Input: dimensioned drawing with shaded views. Units: mm. Origin: part minimum x, y, z. A direction names the side the tool comes from. Coordinates: 2 decimals unless noted, no trailing zeros. Loops run counter-clockwise (first coordinate to the right, second up) from the corner with the lowest first, then second, coordinate; pieces in that order, holes last.
(1) Section C-C, the plane z = 22.5. Return loops of the section in (x, y), then the cut area to 3 significant figures.
(2) Set-up query: the marked faces 5 and 6. Return all of +Z, -Z, +X, -X, +Y, -Y with unobstructed straight access to the full face (end or side cutting, diameter ignored); none if empty.
(3) Section A-A, the plane y = 7. Return loops of the section in (x, z).
(4) Line query: L1, parallel to Y at x = 27.5, z = 11.75; L2, parallel to Z at x = 47, y = 9.5; L3, parallel to Y at x = 45, z = 25.9. Output: solid intervals per line, ascending.
(5) Contact query for flat-ended pins moving along their axis: P1, Ø8, axis at x = 20.5, y = 9.5, coming from the -Z side; P2, Ø4, axis at x = 15.5, y = 12, coming from the -Z side; P3, Ø0.8, axis at x = 7, y = 1, coming from the -Z side; P4, Ø8, axis at x = 25, z = 5, coming from the -Y side. Output: stop coordinate, or through.
(6) Section B-B, the plane x = 5. Return loops of the section in (y, z), then the cut area to 3 significant figures.
(7) Mould query, pull axis Y, two halves, no side actions, for the marked faces 1, 2, 3 and 4. Classes: released by +Y, released by -Y, zero draft, split by the parting line, or undercut.
(8) Section D-D, the plane x = 25. Return loops of the section in (y, z).
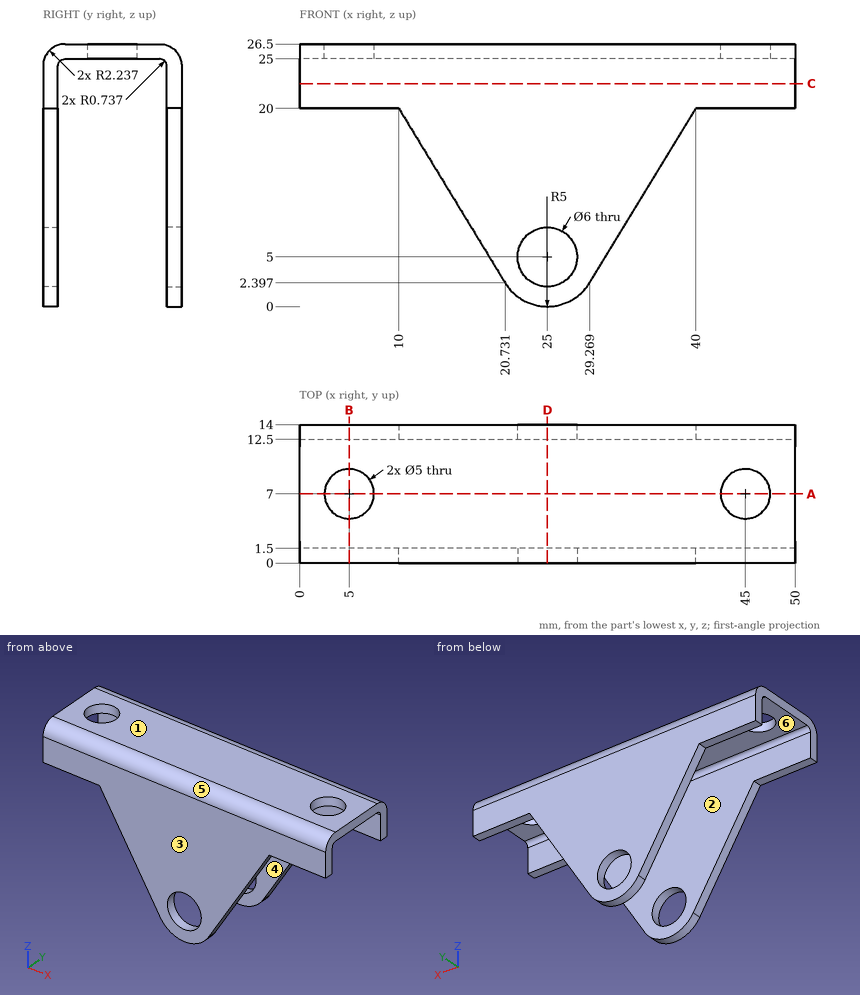
Report:
1. outline: (0, 0) - (50, 0) - (50, 1.5) - (0, 1.5) - close; (0, 12.5) - (50, 12.5) - (50, 14) - (0, 14) - close
1. area: 150 mm2
2. face 5: +Z, +X, -X, -Y
2. face 6: -Z, +X, -X
3. outline: (0, 25) - (2.5, 25) - (2.5, 26.5) - (0, 26.5) - close; (7.5, 25) - (42.5, 25) - (42.5, 26.5) - (7.5, 26.5) - close; (47.5, 25) - (50, 25) - (50, 26.5) - (47.5, 26.5) - close
4. L1: y = 0 to 1.5, 12.5 to 14
4. L2: z = 25 to 26.5
4. L3: y = 0.71 to 4.5, 9.5 to 13.29
5. P1: stops at z = 0.36
5. P2: stops at z = 7.8
5. P3: stops at z = 20
5. P4: stops at y = 0
6. outline: (0, 20) - (1.5, 20) - (1.5, 24.26) arc R0.74 cw to (2.24, 25) - (4.5, 25) - (4.5, 26.5) - (2.24, 26.5) arc R2.24 ccw to (0, 24.26) - close; (9.5, 25) - (11.76, 25) arc R0.74 cw to (12.5, 24.26) - (12.5, 20) - (14, 20) - (14, 24.26) arc R2.24 ccw to (11.76, 26.5) - (9.5, 26.5) - close
6. area: 26.6 mm2
7. face 1: zero draft
7. face 2: undercut
7. face 3: released by -Y
7. face 4: undercut
8. outline: (0, 0) - (1.5, 0) - (1.5, 2) - (0, 2) - close; (0, 8) - (1.5, 8) - (1.5, 24.26) arc R0.74 cw to (2.24, 25) - (11.76, 25) arc R0.74 cw to (12.5, 24.26) - (12.5, 8) - (14, 8) - (14, 24.26) arc R2.24 ccw to (11.76, 26.5) - (2.24, 26.5) arc R2.24 ccw to (0, 24.26) - close; (12.5, 0) - (14, 0) - (14, 2) - (12.5, 2) - close
